Input: part model. Units: mm. Frame: model coordinates. A direction names the side the tool comes from. Round coordinates to 2 decimals unless told otherwise and drop trailing zeros. Loops run counter-clockwise (first coordinate to the right, second up) from the corner with the lowest first, then second, coordinate; pieces in that order, holes last.
(1) Draft query along X for faces 1 (the face through (21.19, -6.261, 86.338)), 2 (the face through (34, 0, 2)), 3 (the face through (42, -6, 44.45)). Return one class per face: released by +X, released by -X, zero draft, split by the parting line, or undercut.
(2) Line query: line 1 (X direction, y = -3.75, z = 70.5); line 2 (Z direction, x = 63.5, y = -11.25); line 3 (X direction, y = -3.25, z = 59). Output: solid intervals per line, ascending.
(3) Cut plane C-C, the plane y = -5.5. Output: boundary loops of the cut face in (x, z).
(4) First-contact query: pin 1 Ø1 at (y, z) = (-9, 33.5) entering from +X; pin 2 Ø1 at (y, z) = (-7, 16.5) entering from +X; pin 3 Ø1.6 at (x, y) = (42, -4.5) entering from +Z. Flat tips, straight axial feed; report the tip coordinate or a pass-through.
(5) Cut plane D-D, the plane x = 19.5. Output: boundary loops of the cut face in (y, z) (3 decimals), and give its area (3 significant figures).
(6) Access query for faces 4 (the face through (40.634, -6, 62)), 5 (the face through (0, -6, 2)), 6 (the face through (61, -6, 57.15)). Directions: +Z, -Z, +X, -X, +Y, -Y. A direction counts if a zero-diameter tool reaches every point of the face in a straight line with its end or side. Return the directions, or none.
(7) Cut plane B-B, the plane z = 65.5. Output: boundary loops of the cut face in (x, y).
(8) Cut plane A-A, the plane x = 66. Output: boundary loops of the cut face in (y, z), and give its area (3 significant figures).
from build123d import *

# Parameters (mm, degrees)
F1_DEPTH = 12.7


with BuildPart() as f1:
    # F0 (on Front) → F1 (new body)
    with BuildSketch(Plane.XZ):
        with BuildLine():
            ThreePointArc((40.634353, 79.069965), (20.903231, 86.407551), (0, 88.9))
            Line((0, 88.9), (0, -87.988181))
            Line((0, -87.988181), (12.7, -87.988181))
            ThreePointArc((12.7, -87.988181), (78.344263, -42.016501), (80.321853, 38.1))
            Line((80.321853, 38.1), (54.921853, 38.1))
            Line((54.921853, 38.1), (54.921853, 57.15))
            Line((54.921853, 57.15), (68.096164, 57.15))
            ThreePointArc((68.096164, 57.15), (56.857557, 68.340532), (43.809353, 77.355999))
            Line((43.809353, 77.355999), (43.809353, 44.45))
            Line((43.809353, 44.45), (40.634353, 44.45))
            Line((40.634353, 44.45), (40.634353, 79.069965))
        make_face()
    extrude(amount=F1_DEPTH)


solid = f1.part
Reported:
1. face 1: released by +X
1. face 2: zero draft
1. face 3: undercut
2. line 1: x = 0 to 40.63, 43.81 to 54.16
2. line 2: z = -62.22 to 38.1, 57.15 to 62.22
2. line 3: x = 0 to 40.63, 43.81 to 66.5
3. outline: (0, -87.99) - (12.7, -87.99) arc R88.9 ccw to (80.32, 38.1) - (54.92, 38.1) - (54.92, 57.15) - (68.1, 57.15) arc R88.9 ccw to (43.81, 77.36) - (43.81, 44.45) - (40.63, 44.45) - (40.63, 79.07) arc R88.9 ccw to (0, 88.9) - close
4. pin 1: stops at x = 82.55
4. pin 2: stops at x = 87.45
4. pin 3: stops at z = 44.45
5. outline: (-12.7, -86.735) - (0, -86.735) - (0, 86.735) - (-12.7, 86.735) - close
5. area: 2,200 mm2
6. face 4: +Z, +Y, -Y
6. face 5: +Z, -Z, -X, +Y, -Y
6. face 6: +X, +Y, -Y
7. outline: (0, -12.7) - (40.63, -12.7) - (40.63, 0) - (0, 0) - close; (43.81, -12.7) - (60.11, -12.7) - (60.11, 0) - (43.81, 0) - close
8. outline: (-12.7, -59.56) - (0, -59.56) - (0, 38.1) - (-12.7, 38.1) - close; (-12.7, 57.15) - (0, 57.15) - (0, 59.56) - (-12.7, 59.56) - close
8. area: 1,270 mm2
